Build history of the part. All positions in model axes, mm. Round coordinates to 2 decimals unless told otherwise and drop trailing zeros. Write each loop counter-clockwise with the first axis right and the second up, starting at its lowest first coordinate (ties: lowest second). Pieces come first, ordered by that corner, then holes. Notation, with made-up numbers: (13.5, 60.25) -> (37.5, 60.25) arc R15 cw to (37.5, 81.25) -> close; hole circle Ø4 at (50.5, 79.5). An arc over 180 degrees is marked (long way). Answer in a Markdown table with one row per item.
```python
from build123d import *

# Parameters (mm, degrees)
SKETCH1_R                                      = 103
BASE_DISC_DEPTH                                = 1.5
SKETCH3_R                                      = 3
CUT_EXTRUDE1_DEPTH                             = 146.671719973
SKETCH4_RX                                     = 28
SKETCH4_RY                                     = 16
CUT_EXTRUDE2_DEPTH                             = 146.671719973
SKETCH2_R                                      = 7.5
CUT_EXTRUDE3_DEPTH                             = 146.671720116
CIRPATTERN3_COUNT                              = 4
CIRPATTERN4_COUNT                              = 4
SKETCH5_R                                      = 1.4
CUT_EXTRUDE4_DEPTH                             = 146.671720116
SKETCH6_R                                      = 7.51
SKETCH6_R_2                                    = 7
CENTRE_BORE_CORRECTION_D14_DEPTH               = 1.5
SKETCH7_R                                      = 5.01
REVB_FOUR_CARTRIDGE_PILOT_HOLES_D10P02_R_DEPTH = 146.671720116


with BuildPart() as part:
    # Sketch1 → Base Disc (new body)
    with BuildSketch(Plane.XY):
        Circle(SKETCH1_R)
    extrude(amount=BASE_DISC_DEPTH)

    # Sketch3 → Cut-Extrude1 (cut, through all)
    with BuildSketch(Plane(origin=(0, 0, 0), x_dir=(-1, 0, 0), z_dir=(0, 0, -1))):
        with Locations((95, 0)):
            Circle(SKETCH3_R)
    cut_extrude1 = extrude(amount=-CUT_EXTRUDE1_DEPTH, mode=Mode.SUBTRACT)

    # Sketch4 → Cut-Extrude2 (cut, through all)
    with BuildSketch(Plane(origin=(0, 0, 0), x_dir=(-1, 0, 0), z_dir=(0, 0, -1))):
        with Locations(Location((38.890872965, 38.890872965), (0, 0, 135))):
            Ellipse(SKETCH4_RX, SKETCH4_RY)
    cut_extrude2 = extrude(amount=-CUT_EXTRUDE2_DEPTH, mode=Mode.SUBTRACT)

    # Sketch2 → Cut-Extrude3 (cut, through all)
    with BuildSketch(Plane(origin=(0, 0, 0), x_dir=(-1, 0, 0), z_dir=(0, 0, -1))):
        Circle(SKETCH2_R)
    extrude(amount=-CUT_EXTRUDE3_DEPTH, mode=Mode.SUBTRACT)

    # CirPattern3: Cut-Extrude1 ×4 about axis
    cirpattern3_axis = Axis((0, 0, 0), (0, 0, 1))
    for i in range(1, CIRPATTERN3_COUNT):
        add(cut_extrude1.rotate(cirpattern3_axis, i * 360 / CIRPATTERN3_COUNT), mode=Mode.SUBTRACT)

    # CirPattern4: Cut-Extrude2 ×4 about axis
    cirpattern4_axis = Axis((0, 0, 0), (0, 0, -1))
    for i in range(1, CIRPATTERN4_COUNT):
        add(cut_extrude2.rotate(cirpattern4_axis, i * 360 / CIRPATTERN4_COUNT), mode=Mode.SUBTRACT)

    # Sketch5 → Cut-Extrude4 (cut, through all)
    with BuildSketch(Plane.XY):
        with Locations((-7.778174593, -7.778174593)):
            Circle(SKETCH5_R)
        with Locations((-7.778174593, 7.778174593)):
            Circle(SKETCH5_R)
        with Locations((7.778174593, 7.778174593)):
            Circle(SKETCH5_R)
        with Locations((7.778174593, -7.778174593)):
            Circle(SKETCH5_R)
    extrude(amount=CUT_EXTRUDE4_DEPTH, mode=Mode.SUBTRACT)

    # Sketch6 → Centre_Bore_Correction_D14 (add)
    with BuildSketch(Plane.XY):
        Circle(SKETCH6_R)
        Circle(SKETCH6_R_2, mode=Mode.SUBTRACT)
    extrude(amount=CENTRE_BORE_CORRECTION_D14_DEPTH)

    # Sketch7 → RevB_Four_Cartridge_Pilot_Holes_D10p02_R95 (cut, through all)
    with BuildSketch(Plane(origin=(0, 0, 0), x_dir=(-1, 0, 0), z_dir=(0, 0, -1))):
        with Locations((-95, 0)):
            Circle(SKETCH7_R)
        with Locations((0, 95)):
            Circle(SKETCH7_R)
        with Locations((95, 0)):
            Circle(SKETCH7_R)
        with Locations((0, -95)):
            Circle(SKETCH7_R)
    extrude(amount=-REVB_FOUR_CARTRIDGE_PILOT_HOLES_D10P02_R_DEPTH, mode=Mode.SUBTRACT)


solid = part.part
```
Q1. Two-plate mould, pull along X, no slides. Class faces 1 (the flat face through (-1, -21, 1.5)), 2 (the cylindrical face through (-2.693, -90.776, 0.74)), 3 (the cylindrical face through (-22.33, -100.55, 0.74)): released by +X, released by -X, zero draft, split by the parting line, or undercut.
A:
| item | result |
|---|---|
| face 1 | zero draft |
| face 2 | undercut |
| face 3 | split by the parting line |
Q2. Saw through at C-C on x = 95. Write the cut outline in (y, z), plus the area to 3 significant figures.
A:
| item | result |
|---|---|
| outline | (-39.8, 0) -> (-5.01, 0) -> (-5.01, 1.5) -> (-39.8, 1.5) -> close; (5.01, 0) -> (39.8, 0) -> (39.8, 1.5) -> (5.01, 1.5) -> close |
| area | 104 mm² |
Q3. Saw through at A-A on x = 0. Write the cut outline in (y, z).
A:
| item | result |
|---|---|
| outline | (-103, 0) -> (-100.01, 0) -> (-100.01, 1.5) -> (-103, 1.5) -> close; (-89.99, 0) -> (-7, 0) -> (-7, 1.5) -> (-89.99, 1.5) -> close; (7, 0) -> (89.99, 0) -> (89.99, 1.5) -> (7, 1.5) -> close; (100.01, 0) -> (103, 0) -> (103, 1.5) -> (100.01, 1.5) -> close |
Q4. Wall check: line 1 (Y direction, x = 0, z = 0.9); line 2 (Y direction, x = 57, z = 0.75); line 3 (X direction, y = -28, z = 0.95). Give the ranges that are in metal, low to high. Write a range as [from, to].
A:
| item | result |
|---|---|
| line 1 | [-103, -100.01], [-89.99, -7], [7, 89.99], [100.01, 103] |
| line 2 | [-85.79, -41.64], [-17.76, 17.76], [41.64, 85.79] |
| line 3 | [-99.12, -61.68], [-27.16, 27.16], [61.68, 99.12] |
